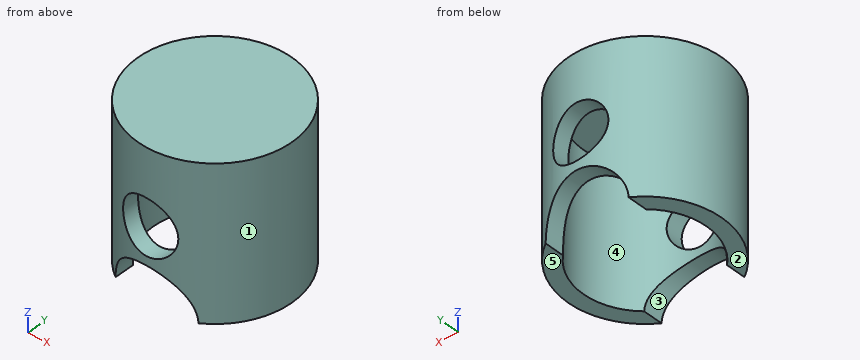
```python
from build123d import *

# Parameters (mm, degrees)
F3_R          = 3.599766951
F4_DEPTH      = 10.001
F4_DEPTH_BACK = 10.001
F6_DEPTH      = 10.0010001
F6_DEPTH_BACK = 10.0010001


with BuildPart() as f2:
    # F0 (on Right) → F2 (revolve)
    with BuildSketch(Plane.YZ):
        Polygon((0, 18), (0, 20), (-10, 20), (-10, 0.1677852448), (-8, 0.1677852448), (-8, 18), align=None)
    revolve(axis=Axis((0, 0, 9.9367983639), (0, 0, -1)))

    # F3 (on Front) → F4 (cut, two sides)
    with BuildSketch(Plane.XZ) as f4_sk:
        with Locations((0, 10.1677852448)):
            Circle(F3_R)
    extrude(amount=-F4_DEPTH, mode=Mode.SUBTRACT)
    extrude(f4_sk.sketch, amount=F4_DEPTH_BACK, mode=Mode.SUBTRACT)

    # F5 (on Front) → F6 (cut, two sides)
    with BuildSketch(Plane.XZ) as f6_sk:
        with BuildLine():
            Line((-5.4118316221, 0), (5.4118316221, 0))
            ThreePointArc((5.4118316221, 0), (0, 5.4118316221), (-5.4118316221, 0))
        make_face()
    extrude(amount=-F6_DEPTH, mode=Mode.SUBTRACT)
    extrude(f6_sk.sketch, amount=F6_DEPTH_BACK, mode=Mode.SUBTRACT)


solid = f2.part
```
Source: CAD feature listing. Evaluate the final solid. Frame: model axes, mm. Face numbers are marked on the shaded views. A direction names the side the tool comes from. Give positions to 0.01 mm unless a question says otherwise; leave off trailing zeros. Loops run counter-clockwise (first coordinate to the right, second up) from the corner with the lowest first, then second, coordinate; pieces in that order, holes last. Notation, with made-up numbers: (-29, 49) -> (24, 49) arc R18 ccw to (24, 78) -> close; hole circle Ø6 at (25, -7.75). An arc over 180 degrees is marked (long way). Use a Markdown table: item, result. Add a question column.
(1) Section query B-B (z = 11.5). Output: boundary loops of the cut face in (x, y).
(2) Section query C-C (y = 0). Output: boundary loops of the cut face in (x, z).
(3) Section query D-D (x = 3). Output: boundary loops of the cut face in (y, z).
(4) Access query for the marked faces 4 and 5. Directions: +Z, -Z, +X, -X, +Y, -Y. A direction counts if a zero-diameter tool reaches every point of the face in a straight line with its end or side. Return the directions, or none.
(5) First-contact query: pin 1 Ø11.5 at (x, z) = (0, 10.17) entering from -Y; pin 2 Ø1.5 at (y, z) = (3.5, 11.5) entering from -X; pin 3 Ø1.5 at (x, y) = (4.5, -2) entering from -Z; pin 4 Ø6.5 at (x, z) = (0, 10.17) entering from +Y. Flat tips, straight axial feed; report the tip coordinate or a pass-through.
(6) Section query A-A (x = 0). Output: boundary loops of the cut face in (y, z).
(7) Ray query, line 1 (Z direction, x = 0, y = -8.75); line 2 (X direction, y = 0, z = 13.5). Return the intervals inside material, ascending.
(8) Pull-direction query (X, two-part tool) for the marked faces 1, 2 and 3; classes: +X half, -X half, draft (parallel to the pull), parting line (faces both ways), or undercut.
Checked values:
| question | item | result |
|---|---|---|
| 1 | outline | (-3.34, -9.42) -> (-3.34, -7.27) arc R8 cw to (-3.34, 7.27) -> (-3.34, 9.42) arc R10 ccw to start; (3.34, -9.42) arc R10 ccw to (3.34, 9.42) -> (3.34, 7.27) arc R8 cw to (3.34, -7.27) -> close |
| 2 | outline | (-10, 0.17) -> (-8, 0.17) -> (-8, 18) -> (8, 18) -> (8, 0.17) -> (10, 0.17) -> (10, 20) -> (-10, 20) -> close |
| 3 | outline | (-9.54, 4.5) -> (-7.42, 4.5) -> (-7.42, 8.18) -> (-9.54, 8.18) -> close; (-9.54, 12.16) -> (-7.42, 12.16) -> (-7.42, 18) -> (7.42, 18) -> (7.42, 12.16) -> (9.54, 12.16) -> (9.54, 20) -> (-9.54, 20) -> close; (7.42, 4.5) -> (9.54, 4.5) -> (9.54, 8.18) -> (7.42, 8.18) -> close |
| 4 | face 4 | -Z |
| 4 | face 5 | -Z, +X, -X, +Y, -Y |
| 5 | pin 1 | y = -10 |
| 5 | pin 2 | x = -9.61 |
| 5 | pin 3 | z = 18 |
| 5 | pin 4 | through |
| 6 | outline | (-10, 5.41) -> (-8, 5.41) -> (-8, 6.57) -> (-10, 6.57) -> close; (-10, 13.77) -> (-8, 13.77) -> (-8, 18) -> (8, 18) -> (8, 13.77) -> (10, 13.77) -> (10, 20) -> (-10, 20) -> close; (8, 5.41) -> (10, 5.41) -> (10, 6.57) -> (8, 6.57) -> close |
| 7 | line 1 | 5.41 to 6.57, 13.77 to 20 |
| 7 | line 2 | -10 to -8, 8 to 10 |
| 8 | face 1 | parting line |
| 8 | face 2 | draft |
| 8 | face 3 | undercut |
